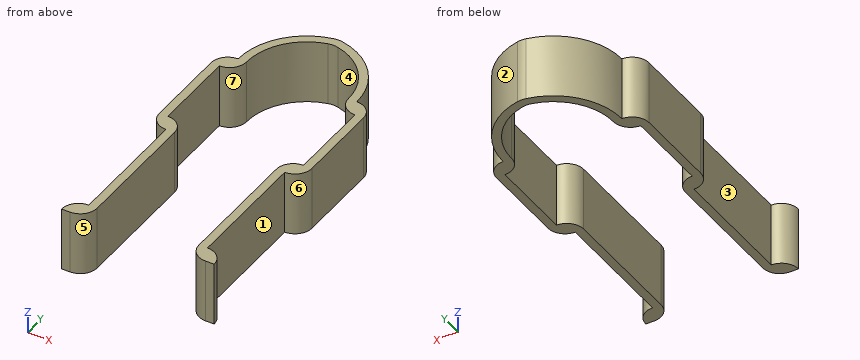
```python
from build123d import *

# Parameters (mm, degrees)
F2_DEPTH = 15
F3_R     = 5


with BuildPart() as f2:
    # F1 (on Top) → F2 (new body)
    with BuildSketch(Plane.XY):
        with BuildLine():
            Line((0, 30), (0, 28))
            ThreePointArc((0, 28), (8.589469, 23.219544), (12, 14))
            ThreePointArc((12, 14), (13.171573, 11.171573), (16, 10))
            Line((16, 10), (16, -10))
            ThreePointArc((16, -10), (13.171573, -11.171573), (12, -14))
            Line((12, -14), (12, -44))
            ThreePointArc((12, -44), (13.171573, -46.828427), (16, -48))
            Line((16, -48), (18, -48))
            ThreePointArc((18, -48), (16.828427, -45.171573), (14, -44))
            Line((14, -44), (14, -14))
            ThreePointArc((14, -14), (16.828427, -12.828427), (18, -10))
            Line((18, -10), (18, 10))
            ThreePointArc((18, 10), (16.828427, 12.828427), (14, 14))
            ThreePointArc((14, 14), (10.107982, 24.521127), (0.305882, 29.976471))
            Line((0.305882, 29.976471), (0, 30))
        make_face()
        with BuildLine():
            Line((-16, -10), (-16, 10))
            ThreePointArc((-16, 10), (-13.171573, 11.171573), (-12, 14))
            ThreePointArc((-12, 14), (-8.589469, 23.219544), (0, 28))
            Line((0, 28), (0, 30))
            Line((0, 30), (-0.305882, 29.976471))
            ThreePointArc((-0.305882, 29.976471), (-10.107982, 24.521127), (-14, 14))
            ThreePointArc((-14, 14), (-16.828427, 12.828427), (-18, 10))
            Line((-18, 10), (-18, -10))
            ThreePointArc((-18, -10), (-16.828427, -12.828427), (-14, -14))
            Line((-14, -14), (-14, -44))
            ThreePointArc((-14, -44), (-16.828427, -45.171573), (-18, -48))
            Line((-18, -48), (-16, -48))
            ThreePointArc((-16, -48), (-13.171573, -46.828427), (-12, -44))
            Line((-12, -44), (-12, -14))
            ThreePointArc((-12, -14), (-13.171573, -11.171573), (-16, -10))
        make_face()
    extrude(amount=F2_DEPTH)

    # F3
    f3_edges = [f2.edges().sort_by_distance(p)[0] for p in [
        (0, 30, 7.5),
        (0, 28, 7.5),
    ]]
    fillet(f3_edges, radius=F3_R)


solid = f2.part
```
Here's how the part is built. I have some questions about the finished solid (model axes, mm). Face numbers are marked on the shaded views. A direction names the side the tool comes from. Give positions to 0.01 mm unless a question says otherwise; leave off trailing zeros. Write each loop counter-clockwise with the first axis right and the second up, starting at its lowest first coordinate (ties: lowest second). Pieces come first, ordered by that corner, then holes. Notation, with made-up numbers: (3, -35.75) -> (11, -35.75) arc R19 cw to (11, -2.75) -> close; hole circle Ø11 at (-17.5, 76). An arc over 180 degrees is marked (long way). Write each question's results on one line, items separated by ' | '.
Item 1: Suppose I cut it at A-A on y = -21. Write out the boundary of the cut face in (x, z), plus the area to 3 significant figures.
Output:
outline: (-14, 0) -> (-12, 0) -> (-12, 15) -> (-14, 15) -> close; (12, 0) -> (14, 0) -> (14, 15) -> (12, 15) -> close | area: 60.0 mm^2
Item 2: Suppose I cut it at C-C on x = -7.5. Write out the boundary of the cut face in (y, z).
Output:
outline: (24.36, 0) -> (26.96, 0) -> (26.96, 15) -> (24.36, 15) -> close
Item 3: For pin 1 Ø4.5 at (y, z) = (-26, 5) entering from +X; pin 2 Ø1.5 at (x, z) = (-13, 10) entering from -Y; pin 3 Ø6 at (x, z) = (4.5, 8.5) entering from +Y, each with a flat end and sliding along its axis, tell me the tip position at first contact or that it passes through.
Output:
pin 1: stops at x = 14 | pin 2: stops at y = -47.31 | pin 3: stops at y = 29.75
Item 4: Suppose I cut it at B-B on x = 13. Write out the boundary of the cut face in (y, z), plus the area to 3 significant figures.
Output:
outline: (-46.65, 0) -> (-11.35, 0) -> (-11.35, 15) -> (-46.65, 15) -> close; (11.35, 0) -> (19.6, 0) -> (19.6, 15) -> (11.35, 15) -> close | area: 653 mm^2
Item 5: Suppose I cut it at D-D on x = 3.5. Write out the boundary of the cut face in (y, z), plus the area to 3 significant figures.
Output:
outline: (26.98, 0) -> (29.14, 0) -> (29.14, 15) -> (26.98, 15) -> close | area: 32.4 mm^2
Item 6: If I drill on L1, parallel to X at y = -19.5, z = 1.75; L2, parallel to X at y = -5, z = 3; L3, parallel to Y at x = 15, z = 4.25, over which ranges is the centre line in solid material (lowest first)?
Output:
L1: x = -14 to -12, 12 to 14 | L2: x = -18 to -16, 16 to 18 | L3: y = -47.87 to -44.13, -13.87 to -10.13, 10.13 to 13.87
Item 7: On a 3-axis mill with a long thin cutter (end or side, diameter ignored), from which of +Z, -Z, +X, -X, +Y, -Y can I reach the whole of each face in a straight line? I mean the marked faces 5, 6 and 7. Say none if no direction works.
Output:
face 5: +Z, -Z, -Y | face 6: +Z, -Z, +X | face 7: +Z, -Z
Item 8: We'd pull the mould along Y, two halves only. Please class the marked faces 1, 2, 3 and 4: pulls with the +Y half, pulls with the -Y half, needs draft (parallel to the pull), parting line crosses it, or undercut.
Output:
face 1: undercut | face 2: pulls with the +Y half | face 3: undercut | face 4: pulls with the -Y half
